Autodesk Inventor part; units mm, degrees
ref_plane "YZ Plane" through (0, 0, 0) normal (1, 0, 0) x (0, 1, 0)
ref_plane "XZ Plane" through (0, 0, 0) normal (0, 1, 0) x (-1, 0, 0)
ref_plane "XY Plane" through (0, 0, 0) normal (0, 0, 1) x (1, 0, 0)
sketch "Sketch1" plane through (0, 0, 0) normal (1, 0, 0) x (0, 1, 0)
  line L0 (0, 22.5) -> (0, -22.5)
  arc A0 (68.1391, -9.7685) -> (68.1391, 9.7685) centre (66, 0) ccw
  line L1 (0, 22.5) -> (10, 22.5)
  line L2 (0, -22.5) -> (10, -22.5)
  line L3 (10, -22.5) -> (68.1391, -9.7685)
  line L4 (10, 22.5) -> (68.1391, 9.7685)
  point P0 (0, 0)
  dimension "d1" = 10
  dimension "d2" = 10
  dimension "d3" = 66
  dimension "d4" = 45
extrude "Extrusion1" add sketch "Sketch1" along normal blind 6
sketch "Sketch2" plane through (6, 0, 0) normal (1, 0, 0) x (0, 0, -1)
  line L0 (-22.5, 0) -> (22.5, 0)
  line L1 (22.5, 10) -> (9.7685, 68.1391)
  line L2 (-9.7685, 68.1391) -> (-22.5, 10)
  line L3 (-11.7222, 45.1931) -> (-19.8985, 7.8557)
  line L4 (-15.9911, 3) -> (15.9911, 3)
  line L5 (19.8985, 7.8557) -> (11.7222, 45.1931)
  arc A0 (11.7222, 45.1931) -> (-11.7222, 45.1931) centre (0, 42.6261) ccw
  arc A1 (-19.8985, 7.8557) -> (-15.9911, 3) centre (-15.9911, 7) ccw
  arc A2 (15.9911, 3) -> (19.8985, 7.8557) centre (15.9911, 7) ccw
  point P0 (0, 0)
  dimension "d8" = 4
  dimension "d9" = 12
  dimension "d10" = 3
  dimension "d11" = 3
  dimension "d12" = 3
extrude "Extrusion2" cut sketch "Sketch2" against normal blind 4
sketch "Sketch3" plane through (6, 0, 0) normal (1, 0, 0) x (0, 0, -1)
  arc A0 (9.7685, 68.1391) -> (-9.7685, 68.1391) centre (0, 66) ccw
  point P0 (0, 0)
hole "Hole1" at (6, 66, 0) direction (-1, 0, 0) diameter 10 end through all
properties part number "Bearing High"
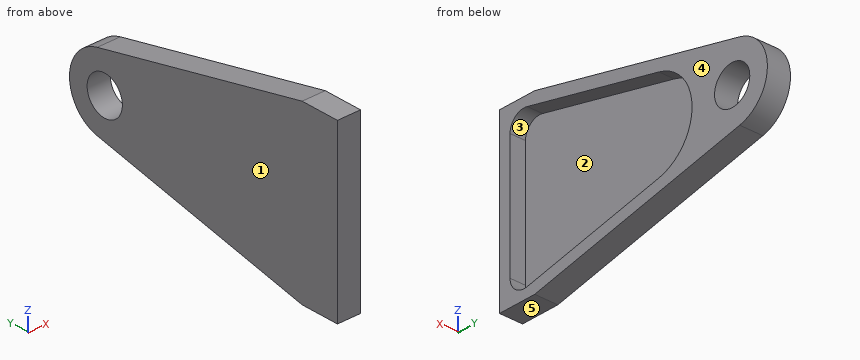
For this review, take the finished solid that the model builds, in its own axes (mm). Face numbers are marked on the shaded views. A direction names the side the tool comes from. Give positions to 0.01 mm unless a question says otherwise; leave off trailing zeros. Write each loop counter-clockwise with the first axis right and the second up, starting at its lowest first coordinate (ties: lowest second). Pieces come first, ordered by that corner, then holes.
Item 1: Take a section at C-C (y = 66). Give the boundary of the cut face in (x, z), and give its area (3 significant figures).
Item 2: Take a section at D-D (z = 14). Give the boundary of the cut face in (x, y), and give its area (3 significant figures).
Item 3: Take a section at A-A (z = 0). Give the boundary of the cut face in (x, y), and give its area (3 significant figures).
Item 4: Take a section at B-B (x = 0.8). Give the boundary of the cut face in (y, z), and give its area (3 significant figures).
Item 5: Wall thickness on probe 1 along Y at (x, z) = (4.3, 0); probe 2 along Y at (x, z) = (0.6, 0); probe 3 along Y at (x, z) = (5.75, 1.5): over which ranges is each line inside the solid? List them lowest first.
Item 6: Insertion check: P1, Ø3, axis at x = 2.5, z = -10.5, coming from the -Y side; P2, Ø1, axis at y = 28, z = -9.5, coming from the +X side. Each pin has a flat end and moves straight along its axis. Give the tip position at first contact, or say it passes through.
Item 7: The part is to be moulded in two halves that separate along Z. For the marked faces 3, 4 and 5, say which applies: +Z half, -Z half, draft (parallel to the pull), parting line (faces both ways), or undercut.
Item 8: Machinability: for the marked faces 1 and 2, which of the approach directions +Z, -Z, +X, -X, +Y, -Y give a long, thin tool a straight path to every point of the face, cutting with its end or side? Answer none if there is none.
Established:
1. outline: (0, -10.24) - (6, -10.24) - (6, -5) - (0, -5) - close; (0, 5) - (6, 5) - (6, 10.24) - (0, 10.24) - close
1. area: 62.8 mm2
2. outline: (0, 0) - (6, 0) - (6, 3) - (2, 3) - (2, 34.79) - (6, 34.79) - (6, 48.82) - (0, 48.82) - close
2. area: 166 mm2
3. outline: (0, 0) - (6, 0) - (6, 3) - (2, 3) - (2, 54.63) - (6, 54.63) - (6, 61) - (0, 61) - close; (0, 71) - (6, 71) - (6, 76) - (0, 76) - close
3. area: 189 mm2
4. outline: (0, -22.5) - (10, -22.5) - (68.14, -9.77) arc R10 ccw to (68.14, 9.77) - (10, 22.5) - (0, 22.5) - close; hole circle Ø10 at (66, 0)
4. area: 2,360 mm2
5. probe 1: y = 0 to 3, 54.63 to 61, 71 to 76
5. probe 2: y = 0 to 61, 71 to 76
5. probe 3: y = 0 to 3, 54.53 to 61.23, 70.77 to 75.89
6. P1: stops at y = 0
6. P2: stops at x = 2
7. face 3: undercut
7. face 4: draft
7. face 5: -Z half
8. face 1: +Z, -Z, -X, +Y, -Y
8. face 2: +X
